The model under review builds one solid part; all positions refer to its coordinate system, in mm. A direction names the side the tool comes from. Round coordinates to 2 decimals unless told otherwise and drop trailing zeros. Order: outer loops, then holes, each group sorted by start corner. A loop starts at its lowest first (then second) coordinate and runs counter-clockwise, first axis right, second up. Notation, with made-up numbers: M -31,-12 L 8,-12 A10 cw 8,-3 Z; hole C 5,25.5 d7. An arc over 180 degrees is marked long. Use a Markdown table: item, result. Add a question column.
1. To check wall thickness, follow probe 1 along X at (y, z) = (25.5, -6.75); probe 2 along Z at (x, y) = (1.25, 15); probe 3 along Z at (x, y) = (-13, 34.5). State the ranges of each line that lie inside material, in increasing order.
2. Consider section A-A on z = 5. State the section outline as (x, y) points, then the cut area to 3 significant figures.
3. Consider section C-C on x = 0.75. State the section outline as (y, z) points.
4. For faces 1 (the flat face through (0, -1, -10.5)), 2 (the flat face through (0, -1, -13)), list the 3-axis set-ups (+Z, -Z, +X, -X, +Y, -Y) from which the entire face can be reached by the end or side of a thin tool; tool diameter is ignored.
5. Consider section B-B on y = 29.5. State the section outline as (x, z) points, then the cut area to 3 significant figures.
from build123d import *

# Parameters (mm, degrees)
F0_W     = 75
F0_H     = 26
F1_DEPTH = 15
F2_R     = 5
F3_T     = -2.5


with BuildPart() as f1:
    # F0 (on Right) → F1 (new body, symmetric)
    with BuildSketch(Plane.YZ):
        Rectangle(F0_W, F0_H)
    extrude(amount=F1_DEPTH, both=True)

    # F2
    f2_edges = [f1.edges().sort_by_distance(p)[0] for p in [
        (15, 0, -13),
        (-15, 0, -13),
    ]]
    fillet(f2_edges, radius=F2_R)

    # F3
    f3_openings = [f1.faces().sort_by_distance(p)[0] for p in [
        (0, 0, 13),
        (0, -37.5, 0.165751),
        (0, 37.5, 0.165751),
    ]]
    offset(amount=F3_T, openings=f3_openings)


solid = f1.part
Answer block:
| question | item | result |
|---|---|---|
| 1 | probe 1 | -15 to -12.5, 12.5 to 15 |
| 1 | probe 2 | -13 to -10.5 |
| 1 | probe 3 | -12 to 13 |
| 2 | outline | M -15,-37.5 L -12.5,-37.5 L -12.5,37.5 L -15,37.5 Z; M 12.5,-37.5 L 15,-37.5 L 15,37.5 L 12.5,37.5 Z |
| 2 | area | 375 mm^2 |
| 3 | outline | M -37.5,-13 L 37.5,-13 L 37.5,-10.5 L -37.5,-10.5 Z |
| 4 | face 1 | +Z, +Y, -Y |
| 4 | face 2 | -Z, +X, -X, +Y, -Y |
| 5 | outline | M -15,-8 A5 ccw -10,-13 L 10,-13 A5 ccw 15,-8 L 15,13 L 12.5,13 L 12.5,-8 A2.5 cw 10,-10.5 L -10,-10.5 A2.5 cw -12.5,-8 L -12.5,13 L -15,13 Z |
| 5 | area | 184 mm^2 |
